Autodesk Inventor part; units mm, degrees
ref_plane "YZ Plane" through (0, 0, 0) normal (1, 0, 0) x (0, 1, 0)
ref_plane "XZ Plane" through (0, 0, 0) normal (0, 1, 0) x (-1, 0, 0)
ref_plane "XY Plane" through (0, 0, 0) normal (0, 0, 1) x (1, 0, 0)
sketch "Sketch1" plane through (0, 0, 0) normal (0, 1, 0) x (-1, 0, 0)
  line L0 (34.29, -26.543) -> (-34.29, -26.543)
  line L1 (-34.29, -26.543) -> (-34.29, 26.543)
  line L2 (-34.29, 26.543) -> (34.29, 26.543)
  line L3 (34.29, 26.543) -> (34.29, -26.543)
  line L4 (34.29, -17.5006) -> (46.3824, -17.5006)
  line L5 (46.3824, -17.5006) -> (46.3824, -5.5118)
  line L6 (46.3824, -5.5118) -> (34.29, -5.5118)
  line L7 (34.29, -5.5118) -> (34.29, -17.5006)
  point P0 (0, 0)
  point P1 (0, -26.543)
  point P2 (34.29, 0)
  dimension "d0" = 68.58
  dimension "d1" = 53.086
  dimension "d2" = 9.0424
  dimension "d3" = 11.9888
extrude "Extrusion1" add sketch "Sketch1" along normal blind 13.3858
sketch "Sketch2" plane through (0, 13.3858, 0) normal (0, 1, 0) x (1, 0, 0)
  circle A0 centre (-19.05, 24.2401) radius 1.5875
  circle A1 centre (31.75, 10.033) radius 1.5875
  circle A2 centre (31.75, -18.923) radius 1.5875
  circle A3 centre (-19.05, -24.003) radius 1.5875
  line L0 (-34.29, 26.543) -> (-34.29, 17.5006)
  line L1 (34.29, -26.543) -> (34.29, 26.543)
  line L2 (34.29, 26.543) -> (-34.29, 26.543)
  line L3 (-34.29, -26.543) -> (34.29, -26.543)
  point P0 (0, 0)
  dimension "d6" = 15.24
  dimension "d7" = 3.175
  dimension "d9" = 16.51
  dimension "d10" = 7.62
  dimension "d11" = 2.54
  dimension "d12" = 50.8
extrude "Extrusion2" cut sketch "Sketch2" against normal blind 13.3858
properties part number "Arduino"
The listing builds one solid part. Answer for the finished solid, in the listing's coordinates (mm). A direction names the side the tool comes from. Give positions to 0.01 mm unless a question says otherwise; leave off trailing zeros. Write each loop counter-clockwise with the first axis right and the second up, starting at its lowest first coordinate (ties: lowest second). Pieces come first, ordered by that corner, then holes. Notation, with made-up numbers: M 36.5,29 L 42.5,29 A22 cw 42.5,35 Z; hole C -5.75,4.25 d2. An arc over 180 degrees is marked long. Write each question's results on one line, items separated by ' | '.
Q1. Section C-C, the plane z = 6 is taken. Write down the section's boundary in (x, y), then the cut area to 3 significant figures.
Output values:
outline: M -34.29,0 L 34.29,0 L 34.29,13.39 L -34.29,13.39 Z | area: 918 mm2
Q2. A tool of negligible diameter and unlimited length cuts with its end or side. For faces 4 (the flat face through (-5, 13.386, 0)), 5 (the flat face through (-40, 7, -5.512)), 6 (the flat face through (-34.29, 7, -22)), from which of +Z, -Z, +X, -X, +Y, -Y can it reach the whole face along a straight path? Write none if from no direction.
Output values:
face 4: +Z, -Z, +X, -X, +Y | face 5: +Z, -X, +Y, -Y | face 6: -Z, -X, +Y, -Y
Q3. For a pull along X with two mould halves and no side action, classify faces 1 (the flat face through (-34.29, 7, 11)), 2 (the flat face through (-5, 0, 0)), 3 (the cylindrical face through (-19.39, 6.79, -22.69)) as released by +X, released by -X, zero draft, split by the parting line, or undercut.
Output values:
face 1: released by -X | face 2: zero draft | face 3: undercut
Q4. Flat-ended cylindrical pins translate along their axes: P1, Ø5, axis at y = 7, z = -1, coming from the -X side; P2, Ø1.9, axis at x = -19.05, z = 24.003, coming from the +Y side; P3, Ø6, axis at x = -37.5, y = 7, coming from the +Z side. Find the tip coordinate at first contact, or state that the pin passes through.
Output values:
P1: x = -34.29 | P2: through | P3: z = -5.51
Q5. Section B-B, the plane y = 2.5 is taken. Count the separate pieces of the cut face and the enclosed holes in it, then the cut area to 3 significant figures.
Output values:
separate pieces: 1 | enclosed holes: 4 | area: 3,750 mm2
Q6. Section A-A, the plane x = 31.75 is taken. Write down the section's boundary in (y, z), then the cut area to 3 significant figures.
Output values:
outline: M 0,-26.54 L 13.39,-26.54 L 13.39,-11.62 L 0,-11.62 Z; M 0,-8.45 L 13.39,-8.45 L 13.39,17.34 L 0,17.34 Z; M 0,20.51 L 13.39,20.51 L 13.39,26.54 L 0,26.54 Z | area: 626 mm2
Q7. Consider L1, parallel to Z at x = 31.75, y = 5.75; L2, parallel to Z at x = -19.05, y = 5; L3, parallel to X at y = 4.5, z = -24. Determine where each line is inside the solid, lowest interval first. Write a range as from..to.
Output values:
L1: -26.54..-11.62, -8.45..17.34, 20.51..26.54 | L2: -26.54..-25.83, -22.65..22.42, 25.59..26.54 | L3: -34.29..-20.62, -17.48..34.29
